The drawing under review shows one solid part. Ordinate dimensions are in mm from its lowest x, y, z. A direction names the side the tool comes from. Coordinates: 2 decimals unless noted, no trailing zeros. Write each loop counter-clockwise with the first axis right and the second up, starting at its lowest first coordinate (ties: lowest second). Pieces come first, ordered by that corner, then holes.
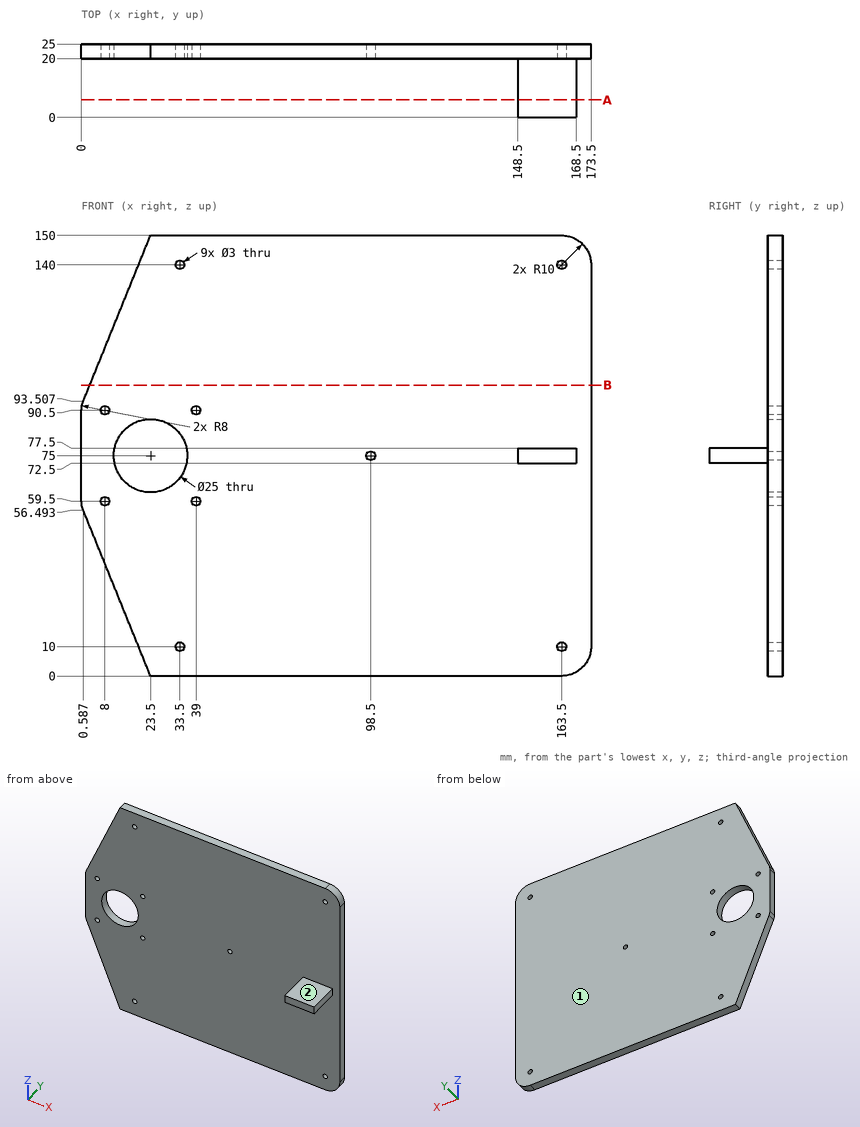
Q1. Add section B-B (z = 99). State the section outline as (x, y) points (1 decimal).
Ans:
outline: (2.8, 20) - (173.5, 20) - (173.5, 25) - (2.8, 25) - close
Q2. Tool access review of the marked faces 1 and 2: name each direction out of +Z, -Z, +X, -X, +Y, -Y from which nothing blocks a thin tool from reaching the whole face with its end or side.
Ans:
face 1: +Z, -Z, +X, -X, +Y
face 2: +Z, +X, -X, -Y
Q3. Clearance check with flat-ended pins moving along their axes: pin 1 Ø10 at (x, y) = (157.5, 8.5) entering from -Z; pin 2 Ø5 at (x, z) = (33.5, 10) entering from -Y; pin 3 Ø4 at (y, z) = (6.5, 74.5) entering from -X. State where each tip first meets the part, or that it passes through.
Ans:
pin 1: stops at z = 72.5
pin 2: stops at y = 20
pin 3: stops at x = 148.5
Q4. For probe 1 along X at (y, z) = (22.1, 90.5); probe 2 along Z at (x, y) = (163.5, 21.4); probe 3 along X at (y, z) = (23.7, 75), list the stretches that pass through material, from the lowest coordinate up.
Ans:
probe 1: x = 0 to 6.5, 9.5 to 37.5, 40.5 to 173.5
probe 2: z = 0 to 8.5, 11.5 to 138.5, 141.5 to 150
probe 3: x = 0 to 11, 36 to 97, 100 to 173.5
Q5. Add section A-A (y = 6). State the section outline as (x, z) points, then the cut area to 3 significant figures.
Ans:
outline: (148.5, 72.5) - (168.5, 72.5) - (168.5, 77.5) - (148.5, 77.5) - close
area: 100 mm2
